```python
from build123d import *

# Parameters (mm, degrees)
CROQUIS1_R              = 1.5
CROQUIS1_R_2            = 4
SALIENTE_EXTRUIR1_DEPTH = 6
CROQUIS4_R              = 4
SALIENTE_EXTRUIR3_DEPTH = 6
CORTAR_EXTRUIR1_DEPTH   = 6
REDONDEO3_R             = 4
CORTAR_EXTRUIR2_DEPTH   = 6
REDONDEO4_R             = 2.5
REDONDEO6_R             = 10


with BuildPart() as part:
    # Croquis1 → Saliente-Extruir1 (new body)
    with BuildSketch(Plane.XY):
        with BuildLine():
            Line((-17.112213819, 2.294275414), (-30.516043414, 23.123582692))
            ThreePointArc((-30.516043414, 23.123582692), (-31.14080226, 23.989156666), (-31.854269143, 24.783201331))
            Line((-31.854269143, 24.783201331), (-45.961940777, 38.890872965))
            Line((-45.961940777, 38.890872965), (-104.121735922, 79.614799946))
            Line((-104.121735922, 79.614799946), (-98.473110707, 87.681872787))
            Line((-98.473110707, 87.681872787), (-38.890872965, 45.961940777))
            Line((-38.890872965, 45.961940777), (-24.783201331, 31.854269143))
            ThreePointArc((-24.783201331, 31.854269143), (-23.989156666, 31.14080226), (-23.123582692, 30.516043414))
            Line((-23.123582692, 30.516043414), (-2.294275414, 17.112213819))
            ThreePointArc((-2.294275414, 17.112213819), (-0.610887166, 15.302496804), (0, 12.907567049))
            Line((0, 12.907567049), (0, 7.055686841))
            ThreePointArc((0, 7.055686841), (-0.823113423, 5.438609853), (-2.614937985, 5.15257064))
            Line((-2.614937985, 5.15257064), (-4.503911831, 5.762938925))
            ThreePointArc((-4.503911831, 5.762938925), (-5.518487605, 5.518487605), (-5.762938925, 4.503911831))
            Line((-5.762938925, 4.503911831), (-5.15257064, 2.614937985))
            ThreePointArc((-5.15257064, 2.614937985), (-5.438609853, 0.823113423), (-7.055686841, 0))
            Line((-7.055686841, 0), (-12.907567049, 0))
            ThreePointArc((-12.907567049, 0), (-15.302496804, 0.610887166), (-17.112213819, 2.294275414))
        make_face()
        with Locations((-38.890872965, 38.890872965)):
            Circle(CROQUIS1_R, mode=Mode.SUBTRACT)
        with Locations((-24.04163056, 24.04163056)):
            Circle(CROQUIS1_R, mode=Mode.SUBTRACT)
        with Locations((-15.25, 15.25)):
            Circle(CROQUIS1_R_2, mode=Mode.SUBTRACT)
    extrude(amount=SALIENTE_EXTRUIR1_DEPTH)

    # Croquis4 → Saliente-Extruir3 (add)
    with BuildSketch(Plane.XY.offset(6)):
        Polygon((-98.473110707, 87.681872787), (-100.447042684, 98.87659732), (-116.83008357, 110.348126047), (-134.88265713, 107.164970257), (-131.69950134, 89.112396696), (-115.316460454, 77.640867969), (-104.121735922, 79.614799946), align=None)
        with Locations((-116.861312156, 94.546288657)):
            Circle(CROQUIS4_R, mode=Mode.SUBTRACT)
    extrude(amount=-SALIENTE_EXTRUIR3_DEPTH)

    # Croquis5 → Cortar-Extruir1 (cut)
    with BuildSketch(Plane.XY.offset(6)):
        with BuildLine():
            Line((-129.005623724, 100.303084339), (-126.548167592, 98.58235503))
            ThreePointArc((-126.548167592, 98.58235503), (-123.41452851, 99.134900148), (-123.967073628, 102.26853923))
            Line((-123.967073628, 102.26853923), (-126.424529761, 103.989268539))
            ThreePointArc((-126.424529761, 103.989268539), (-129.558168842, 103.436723421), (-129.005623724, 100.303084339))
        make_face()
        with BuildLine():
            Line((-116.992750408, 86.653556305), (-116.645454053, 84.683940799))
            ThreePointArc((-116.645454053, 84.683940799), (-114.907770157, 83.467201436), (-113.691030794, 85.204885332))
            Line((-113.691030794, 85.204885332), (-114.038327149, 87.174500838))
            ThreePointArc((-114.038327149, 87.174500838), (-115.776011045, 88.391240201), (-116.992750408, 86.653556305))
        make_face()
        with BuildLine():
            Line((-108.968579803, 94.414850405), (-106.998964297, 94.76214676))
            ThreePointArc((-106.998964297, 94.76214676), (-105.782224934, 96.499830656), (-107.51990883, 97.716570019))
            Line((-107.51990883, 97.716570019), (-109.489524336, 97.369273664))
            ThreePointArc((-109.489524336, 97.369273664), (-110.706263699, 95.631589768), (-108.968579803, 94.414850405))
        make_face()
        with BuildLine():
            Line((-124.754044508, 94.67772691), (-126.723660014, 94.330430555))
            ThreePointArc((-126.723660014, 94.330430555), (-127.940399377, 92.592746659), (-126.202715481, 91.376007296))
            Line((-126.202715481, 91.376007296), (-124.233099975, 91.723303651))
            ThreePointArc((-124.233099975, 91.723303651), (-123.016360612, 93.460987547), (-124.754044508, 94.67772691))
        make_face()
        with BuildLine():
            Line((-116.729873903, 102.43902101), (-117.077170259, 104.408636516))
            ThreePointArc((-117.077170259, 104.408636516), (-118.814854155, 105.625375879), (-120.031593518, 103.887691983))
            Line((-120.031593518, 103.887691983), (-119.684297162, 101.918076477))
            ThreePointArc((-119.684297162, 101.918076477), (-117.946613266, 100.701337114), (-116.729873903, 102.43902101))
        make_face()
    extrude(amount=-CORTAR_EXTRUIR1_DEPTH, mode=Mode.SUBTRACT)

    # Redondeo3
    redondeo3_edges = [part.edges().sort_by_distance(p)[0] for p in [
        (-134.88265713, 107.164970257, 3),
    ]]
    fillet(redondeo3_edges, radius=REDONDEO3_R)

    # Croquis7 → Cortar-Extruir2 (cut)
    with BuildSketch(Plane.XY.offset(6)):
        with BuildLine():
            Line((-131.69950134, 89.112396696), (-115.316460454, 77.640867969))
            ThreePointArc((-115.316460454, 77.640867969), (-122.523879314, 84.782075048), (-131.69950134, 89.112396696))
        make_face()
        with BuildLine():
            Line((-116.83008357, 110.348126047), (-100.447042684, 98.87659732))
            ThreePointArc((-100.447042684, 98.87659732), (-109.62266471, 103.206918969), (-116.83008357, 110.348126047))
        make_face()
    extrude(amount=-CORTAR_EXTRUIR2_DEPTH, mode=Mode.SUBTRACT)

    # Redondeo4
    redondeo4_edges = [part.edges().sort_by_distance(p)[0] for p in [
        (-115.316460454, 77.640867969, 3),
        (-131.69950134, 89.112396696, 3),
        (-116.83008357, 110.348126047, 3),
        (-100.447042684, 98.87659732, 3),
    ]]
    fillet(redondeo4_edges, radius=REDONDEO4_R)

    # Redondeo6
    redondeo6_edges = [part.edges().sort_by_distance(p)[0] for p in [
        (-38.890872965, 45.961940777, 3),
        (-45.961940777, 38.890872965, 3),
        (-104.121735922, 79.614799946, 3),
        (-98.473110707, 87.681872787, 3),
    ]]
    fillet(redondeo6_edges, radius=REDONDEO6_R)


solid = part.part
```
Check sheet for the modelled part. Datum: model origin and axes. Units: mm. A direction names the side the tool comes from. Round coordinates to 2 decimals unless told otherwise and drop trailing zeros. Order: outer loops, then holes, each group sorted by start corner. A loop starts at its lowest first (then second) coordinate and runs counter-clockwise, first axis right, second up.
1) Section check C-C (z = 4.45). Give the number of separate pieces and of enclosed holes in the cut face, and give its area (3 significant figures).
2) Section check D-D (y = 50). Record the boundary of the cut face in (x, z), and give its area (3 significant figures).
3) Tool access check on faces 4 (the cylindrical face through (-115.743, 88.397, 3.042)), 5 (the flat face through (-111, 78.4, 3)), 6 (the cylindrical face through (-5.423, 0.845, 2.958)). Record the directions out of +Z, -Z, +X, -X, +Y, -Y that give a thin tool (end or side, any length) a straight path to the whole face; none if there is none.
4) Mould release check, pull along Y, two halves, no side actions. Record for faces 1 (the cylindrical face through (-40, 39.9, 3)), 2 (the flat face through (-38.5, 31.43, 2.96)), 3 (the flat face through (-72, 59, 6)): +Y half, -Y half, draft (parallel to the pull), parting line (faces both ways), or undercut.
5) Go/stop test with flat-tipped pins: pin 1 Ø7 at (x, y) = (-116.86, 94.55) entering from +Z; pin 2 Ø3.5 at (x, y) = (-24.04, 24.04) entering from -Z; pin 3 Ø1.5 at (y, z) = (81, 3) entering from +X. Record where each tip stops, or that it passes through.
6) Section check A-A (x = -15.25). Record the boundary of the cut face in (y, z), and give its area (3 significant figures).
7) Scan lines: line 1 (X direction, y = 96, z = 2.05); line 2 (X direction, y = 15, z = 3.5); line 3 (Y direction, x = -15.25, z = 3.75). Record each from-to range of solid material in increasing order.
8) Section check B-B (y = 15.25). Record the boundary of the cut face in (x, z), and give its area (3 significant figures).
Result:
1. separate pieces: 1
1. enclosed holes: 9
1. area: 2,040 mm2
2. outline: (-61.83, 0) - (-44.66, 0) - (-44.66, 6) - (-61.83, 6) - close
2. area: 103 mm2
3. face 4: +Z, -Z
3. face 5: +Z, -Z, -Y
3. face 6: +Z, -Z, +X
4. face 1: undercut
4. face 2: -Y half
4. face 3: draft
5. pin 1: passes through
5. pin 2: stops at z = 0
5. pin 3: stops at x = -87.86
6. outline: (0.58, 0) - (11.25, 0) - (11.25, 6) - (0.58, 6) - close; (19.25, 0) - (25.45, 0) - (25.45, 6) - (19.25, 6) - close
6. area: 101 mm2
7. line 1: x = -132.91 to -120.59, -113.13 to -110.73, -105.78 to -99.94
7. line 2: x = -25.29 to -19.24, -11.26 to -0.46
7. line 3: y = 0.58 to 11.25, 19.25 to 25.45
8. outline: (-25.45, 0) - (-19.25, 0) - (-19.25, 6) - (-25.45, 6) - close; (-11.25, 0) - (-0.58, 0) - (-0.58, 6) - (-11.25, 6) - close
8. area: 101 mm2
